Here's how the part is built. I have some questions about the finished solid (model axes, mm). A direction names the side the tool comes from. Round coordinates to 2 decimals unless told otherwise and drop trailing zeros. Write each loop counter-clockwise with the first axis right and the second up, starting at its lowest first coordinate (ties: lowest second). Pieces come first, ordered by that corner, then holes. Notation, with made-up numbers: (-37.5, -27.5) -> (-24.5, -27.5) arc R7 ccw to (-24.5, -21.5) -> close; hole circle Ø9 at (-12.75, 6.25). An arc over 180 degrees is marked (long way). Put each result on its own line as item: value. Start each with the question number.
1) Which directions (+Z, -Z, +X, -X, +Y, -Y) give clear straight access to the entire face, cutting with the end or side of a thin tool? Please do faces 1 (the cylindrical face through (-11.082, -0.811, 7.984)), 2 (the flat face through (10, -1.6, 0)).
2) I want a section at C-C, the plane x = 14.5. List the corners of the cut face in (y, z) for me.
3) I want a section at B-B, the plane z = -13.65. List the corners of the cut face in (x, y) for me (3 decimals), then the cut area to 3 significant figures.
4) I want a section at D-D, the plane y = -0.8. List the corners of the cut face in (x, z) for me (3 decimals).
5) We'd pull the mould along Z, two halves only. Please class faces 3 (the cylindrical face through (17.28, -0.81, -8.27)), 4 (the flat face through (0, -1.9, 0)), 5 (the cylindrical face through (-1.73, -1.75, -7.81)): released by +Z, released by -Z, zero draft, split by the parting line, or undercut.
6) Will these pins go through, and if not, where does the flat tip stop? P1, Ø1, axis at y = -0.5, z = -13, coming from the -X side; P2, Ø2.5, axis at x = -15.37, z = -8.88, coming from the -Y side; P3, Ø6.5, axis at x = 0, z = 17.75, coming from the -Y side.
7) I want a section at A-A, the plane x = 0. List the corners of the cut face in (y, z) for me (3 decimals), then the cut area to 3 significant figures.
8) If I drill on line 1 along Z through (x, y) = (0, -1.2) (3 decimals); line 2 along Y through (x, z) = (15.5, -13); line 3 along Z through (x, y) = (15, -0.1), over which ranges is the centre line in solid material (lowest first)? Write a range as [from, to].
from build123d import *

# Parameters (mm, degrees)
F0_R     = 22.5
F1_DEPTH = 1.6
F2_R     = 8
F3_DEPTH = 0.3
F5_D     = 4
F7_D     = 2.75


with BuildPart() as f1:
    # F0 (on Front) → F1 (new body)
    with BuildSketch(Plane.XZ):
        Circle(F0_R)
    extrude(amount=F1_DEPTH)

    # F2 (on face) → F3 (join)
    with BuildSketch(Plane.XZ.offset(1.6)):
        Circle(F2_R)
    extrude(amount=F3_DEPTH)

    # F5 (through all)
    with Locations(Plane(origin=(0, 0, 0), x_dir=(-1, 0, 0), z_dir=(0, 1, 0))):
        with Locations((0, 17.75), (-15.371951, -8.875), (15.371951, -8.875)):
            Hole(F5_D / 2)

    # F7 (through all)
    with Locations(Plane(origin=(0, 0, 0), x_dir=(-1, 0, 0), z_dir=(0, 1, 0))):
        with Locations((11.821247, 6.825), (0, -13.65), (-11.821247, 6.825)):
            Hole(F7_D / 2)


solid = f1.part
Findings:
1. face 1: +Y, -Y
1. face 2: -Y
2. outline: (-1.6, -17.2) -> (0, -17.2) -> (0, -10.67) -> (-1.6, -10.67) -> close; (-1.6, -7.08) -> (0, -7.08) -> (0, 17.2) -> (-1.6, 17.2) -> close
3. outline: (-17.887, -1.6) -> (-1.375, -1.6) -> (-1.375, 0) -> (-17.887, 0) -> close; (1.375, -1.6) -> (17.887, -1.6) -> (17.887, 0) -> (1.375, 0) -> close
3. area: 52.8 mm2
4. outline: circle Ø45 at (0, 0); hole circle Ø4 at (-15.372, -8.875); hole circle Ø2.75 at (-11.821, 6.825); hole circle Ø4 at (0, 17.75); hole circle Ø2.75 at (0, -13.65); hole circle Ø2.75 at (11.821, 6.825); hole circle Ø4 at (15.372, -8.875)
5. face 3: undercut
5. face 4: zero draft
5. face 5: split by the parting line
6. P1: stops at x = -18.71
6. P2: passes through
6. P3: stops at y = -1.6
7. outline: (-1.9, -8) -> (-1.6, -8) -> (-1.6, -12.275) -> (0, -12.275) -> (0, 15.75) -> (-1.6, 15.75) -> (-1.6, 8) -> (-1.9, 8) -> close; (-1.6, -22.5) -> (0, -22.5) -> (0, -15.025) -> (-1.6, -15.025) -> close; (-1.6, 19.75) -> (0, 19.75) -> (0, 22.5) -> (-1.6, 22.5) -> close
7. area: 66.0 mm2
8. line 1: z = [-22.5, -15.025], [-12.275, 15.75], [19.75, 22.5]
8. line 2: y = [-1.6, 0]
8. line 3: z = [-16.77, -10.84], [-6.91, 16.77]
